from build123d import *

# Parameters (mm, degrees)
F2_SIZE = 0.3


with BuildPart() as f1:
    # F0 (on Front) → F1 (revolve)
    with BuildSketch(Plane.XZ):
        Polygon((6.3, 1.2), (6.3, 0), (9, 0), (9.2, 4.1), (7.741463, 4.1), (7.6, 1.2), align=None)
    revolve(axis=Axis((0, 0, 3.37447), (0, 0, -1)))

    # F2
    f2_edges = [f1.edges().sort_by_distance(p)[0] for p in [
        (-9, 0, 0),
    ]]
    chamfer(f2_edges, length=F2_SIZE)


solid = f1.part
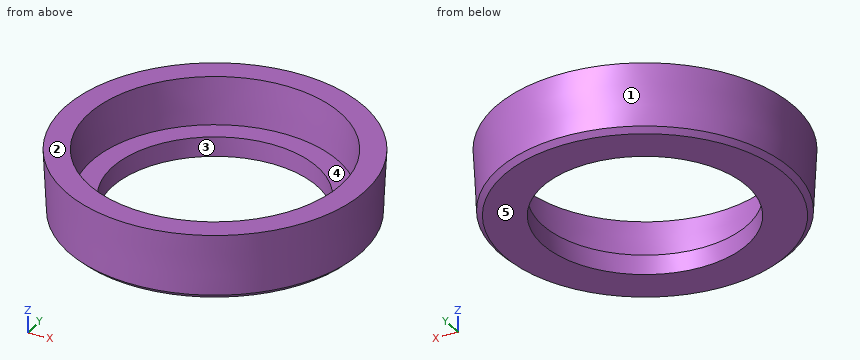
Design review of the part built by this model. Coordinates are the model's own, in mm. Face numbers are marked on the shaded views. A direction names the side the tool comes from. Round coordinates to 2 decimals unless told otherwise and drop trailing zeros. Loops run counter-clockwise (first coordinate to the right, second up) from the corner with the lowest first, then second, coordinate; pieces in that order, holes last. Notation, with made-up numbers: M 22.5,-17 L 79.5,-17 A14 ccw 79.5,-9 Z; hole C 64,0.5 d9. An arc over 180 degrees is marked long. Answer as a JSON object with one key per item and string values.
Item 1: We need section A-A on y = 0. Give the boundary of the cut face in (x, z).
Answer sheet:
{"outline": "M -9.2,4.1 L -9.01,0.3 L -8.7,0 L -6.3,0 L -6.3,1.2 L -7.6,1.2 L -7.74,4.1 Z; M 6.3,0 L 8.7,0 L 9.01,0.3 L 9.2,4.1 L 7.74,4.1 L 7.6,1.2 L 6.3,1.2 Z"}
Item 2: The part is to be moulded in two halves that separate along Y. For the marked faces 1, 2 and 3, say which applies: pulls with the +Y half, pulls with the -Y half, needs draft (parallel to the pull), parting line crosses it, or undercut.
Answer sheet:
{"face 1": "parting line crosses it", "face 2": "needs draft", "face 3": "undercut"}
Item 3: We need section D-D on z = 1.9. Give the boundary of the cut face in (x, y), and give its area (3 significant figures).
Answer sheet:
{"outline": "C 0,0 d18.19; hole C 0,0 d15.27", "area": "76.6 mm^2"}
Item 4: We need section C-C on z = 2.9. Give the boundary of the cut face in (x, y), and give its area (3 significant figures).
Answer sheet:
{"outline": "C 0,0 d18.28; hole C 0,0 d15.37", "area": "77.1 mm^2"}
Item 5: Clearance check with flat-ended pins moving along their axes: P1, Ø2, axis at x = 2, y = 6, coming from the +Z side; P2, Ø1, axis at y = 1.5, z = 1.5, coming from the +X side. State where each tip first meets the part, or that it passes through.
Answer sheet:
{"P1": "stops at z = 1.2", "P2": "stops at x = 9.02"}
Item 6: Wall thickness on L1, parallel to Y at x = 0, z = 0.4; L2, parallel to Y at x = 0.5, z = 3.4; L3, parallel to X at y = 0.5, z = 1.65: over which ranges is each line inside the solid? List them lowest first. Write a range as from..to.
Answer sheet:
{"L1": "y = -9.02..-6.3, 6.3..9.02", "L2": "y = -9.15..-7.69, 7.69..9.15", "L3": "x = -9.07..-7.61, 7.61..9.07"}
Item 7: Machinability: for the marked faces 4 and 5, which of the approach directions +Z, -Z, +X, -X, +Y, -Y give a long, thin tool a straight path to every point of the face, cutting with its end or side? Answer none if there is none.
Answer sheet:
{"face 4": "+Z", "face 5": "-Z, +X, -X, +Y, -Y"}
